from build123d import *

# Parameters (mm, degrees)
F0_W     = 50
F0_H     = 20
F1_DEPTH = 3
F2_R     = 5
F3_DEPTH = 40
F4_W     = 5
F4_H     = 10.295372
F5_DEPTH = 3.001


with BuildPart() as f1:
    # F0 (on Front) → F1 (new body)
    with BuildSketch(Plane.XZ):
        Rectangle(F0_W, F0_H)
    extrude(amount=F1_DEPTH)

    # F2 (on face) → F3 (join)
    with BuildSketch(Plane.XZ.offset(3)):
        with Locations((20, 0)):
            Circle(F2_R)
    extrude(amount=F3_DEPTH)

    # F4 (on face) → F5 (cut, through all)
    with BuildSketch(Plane.XZ.offset(3)):
        with Locations((-17.5, -5.147686)):
            Rectangle(F4_W, F4_H)
    extrude(amount=-F5_DEPTH, mode=Mode.SUBTRACT)


solid = f1.part
Geometry: final body of the model. Coordinates: model frame, mm. A direction names the side the tool comes from. Give positions to 0.01 mm unless a question says otherwise; leave off trailing zeros. Order: outer loops, then holes, each group sorted by start corner. A loop starts at its lowest first (then second) coordinate and runs counter-clockwise, first axis right, second up. Notation, with made-up numbers: (-28.75, -28) -> (21.25, -28) arc R28 cw to (21.25, 6) -> close; hole circle Ø3 at (-13.5, 17). An arc over 180 degrees is marked (long way). Answer as a JSON object with one key per item and string values.
Q1. Material intervals for probe 1 along Y at (x, z) = (13.5, -5.5); probe 2 along X at (y, z) = (-9, -2); probe 3 along X at (y, z) = (-24.5, -1.75), sorted ascending.
Entries:
{"probe 1": "y = -3 to 0", "probe 2": "x = 15.42 to 24.58", "probe 3": "x = 15.32 to 24.68"}
Q2. Draft query along X for faces 3 (the flat face through (0, 0, 0)), 4 (the flat face through (-18, -2, 0)), 5 (the flat face through (-15, -2, -5)), 6 (the cylindrical face through (15, -23, 0)). Return one class per face: released by +X, released by -X, zero draft, split by the parting line, or undercut.
Entries:
{"face 3": "zero draft", "face 4": "undercut", "face 5": "undercut", "face 6": "split by the parting line"}
Q3. Access query for faces 1 (the flat face through (-20, -2, -5)), 2 (the flat face through (-23, -1, -10)). Directions: +Z, -Z, +X, -X, +Y, -Y. A direction counts if a zero-diameter tool reaches every point of the face in a straight line with its end or side. Return the directions, or none.
Entries:
{"face 1": "-Z, +Y, -Y", "face 2": "-Z, +X, -X, +Y, -Y"}
Q4. Section C-C (z = 2.5). Output: boundary loops of the cut face in (x, y), plus the area to 3 significant figures.
Entries:
{"outline": "(-25, -3) -> (15.67, -3) -> (15.67, -43) -> (24.33, -43) -> (24.33, -3) -> (25, -3) -> (25, 0) -> (-25, 0) -> close", "area": "496 mm^2"}
Q5. First-contact query: pin 1 (12 mm diameter, centred on x = -1, z = -5, fed in from -Y); pin 2 (10 mm diameter, centred on y = -6, z = 8, fed in from -X); pin 3 (2 mm diameter, centred on y = -11, z = 1, fed in from -X); pin 4 (3.5 mm diameter, centred on x = -18, y = -1.5, fed in from -Z). Flat tips, straight axial feed; report the tip coordinate or a pass-through.
Entries:
{"pin 1": "stops at y = -3", "pin 2": "stops at x = -25", "pin 3": "stops at x = 15", "pin 4": "stops at z = 0"}
Q6. Section A-A (z = -3). Output: boundary loops of the cut face in (x, y).
Entries:
{"outline": "(-25, -3) -> (-20, -3) -> (-20, 0) -> (-25, 0) -> close; (-15, -3) -> (16, -3) -> (16, -43) -> (24, -43) -> (24, -3) -> (25, -3) -> (25, 0) -> (-15, 0) -> close"}
Q7. Section B-B (x = 20). Output: boundary loops of the cut face in (y, z), plus the area to 3 significant figures.
Entries:
{"outline": "(-43, -5) -> (-3, -5) -> (-3, -10) -> (0, -10) -> (0, 10) -> (-3, 10) -> (-3, 5) -> (-43, 5) -> close", "area": "460 mm^2"}
Q8. Section D-D (y = -14.5). Output: boundary loops of the cut face in (x, z), plus the area to 3 significant figures.
Entries:
{"outline": "circle Ø10 at (20, 0)", "area": "78.5 mm^2"}
